Read the model definition and answer for the solid it produces. Units are mm, in the model's axes. A direction names the side the tool comes from. Coordinates: 2 decimals unless noted, no trailing zeros. Write each loop counter-clockwise with the first axis right and the second up, starting at its lowest first coordinate (ties: lowest second). Pieces come first, ordered by that corner, then holes. Notation, with made-up numbers: (76.5, -23.5) -> (89.5, -23.5) arc R25 cw to (89.5, 4.5) -> close; hole circle Ø8 at (38.5, -14). An arc over 180 degrees is marked (long way). Return JSON: item names as keys, results as strings.
from build123d import *

# Parameters (mm, degrees)
F0_W         = 51.3733290136
F0_H         = 51.9489385188
F1_DEPTH     = 63.5
F3_DEPTH     = 3.556
F4_T         = 2.54
F4_T3_DEPTH  = 13.7734491992
F4_T5_DEPTH  = 11.8834199066
F4_T7_DEPTH  = 11.0801313686
F4_T9_DEPTH  = 13.5809922736
F4_T11_DEPTH = 10.8262574938
F4_T13_DEPTH = 5.3370977176
F5_T1_DEPTH  = 76.2
F6_R         = 5.08


# Not quite as in the source:
# - a fillet or chamfer that OpenCascade refuses, or shapes differently, is made with other operations: its cross-section is extruded or revolved along the edge and cut away or added
# - a shell that OpenCascade refuses in one call is made with other operations: the cavity is built on its own and cut out


with BuildPart() as f1:
    # F0 (on Top) → F1 (new body)
    with BuildSketch(Plane.XY):
        with Locations((-25.6866645068, 25.9744692594)):
            Rectangle(F0_W, F0_H)
    extrude(amount=F1_DEPTH)

    # F2 (on Top) → F3 (join)
    with BuildSketch(Plane.XY):
        Polygon((-51.6957342625, 3.4017099533), (-51.6957342625, 0), (-45.3731976449, 0), (-45.3731976449, 6.8034199066), (-51.6957342625, 6.8034199066), align=None)
        Polygon((-45.3731976449, 43.2554893196), (-45.3731976449, 51.7564815932), (-51.6957342625, 51.9683584571), (-51.6957342625, 47.6119238883), (-51.6957342625, 43.2554893196), align=None)
    extrude(amount=-F3_DEPTH)

    # F4: shell of thickness 2.54, made by hand


with BuildPart() as f4_core1:
    # F4_t2: copy of F1
    add(f1.part)

    # the walls: a layer under each face that stays
    f4_faces = [f4_core1.faces().sort_by_distance(p)[0] for p in [
        (-25.8478671312, 0, 29.972),
        (-51.3733290136, 25.9744692594, 31.75),
        (-25.6866645068, 25.9744692594, 0),
        (-25.6866645068, 25.9744692594, 63.5),
        (-25.6866645068, 51.9489385188, 31.75),
        (-51.4059827792, 47.6119238883, 0),
        (-51.534531638, 3.4017099533, 0),
        (-51.6957342625, 3.4017099533, -1.778),
        (-45.3731976449, 3.4017099533, -1.778),
        (-48.5344659537, 3.4017099533, -3.556),
        (-48.5344659537, 6.8034199066, -1.778),
        (-48.5344659537, 43.2554893196, -1.778),
        (-45.3731976449, 47.5059854564, -1.778),
        (-48.5344659537, 51.8624200251, -1.778),
        (-51.6957342625, 47.6119238883, -1.778),
        (-48.5344659537, 47.6119238883, -3.556),
    ]]
    thicken(f4_faces, amount=-F4_T, mode=Mode.SUBTRACT)

    # F4_s4 → F4_t3 (cut)
    with BuildSketch(Plane.XZ.offset(-54.4889385188)):
        Polygon((-51.3987290136, 0.0254), (-48.8333290136, 0), (-48.8333290136, -2.54), (-51.3733290136, -2.54), align=None)
    extrude(amount=F4_T3_DEPTH, mode=Mode.SUBTRACT)

    # F4_s6 → F4_t5 (cut)
    with BuildSketch(Plane.XZ.offset(-9.3434199066)):
        Polygon((-51.3987290136, 0.0254), (-48.8333290136, 0), (-48.8333290136, -2.54), (-51.3733290136, -2.54), align=None)
        Polygon((-45.3477976449, -0.0254), (-45.3731976449, 2.54), (-47.9131976449, 2.54), (-47.9131976449, 0), align=None)
    extrude(amount=F4_T5_DEPTH, mode=Mode.SUBTRACT)

    # F4_s8 → F4_t7 (cut)
    with BuildSketch(Plane.YZ.offset(-53.9133290136)):
        Polygon((6.8288199066, -0.0254), (6.8034199066, 2.54), (4.2634199066, 2.54), (4.2634199066, 0), align=None)
        Polygon((43.2300893196, -0.0254), (43.2554893196, 2.54), (45.7954893196, 2.54), (45.7954893196, 0), align=None)
    extrude(amount=F4_T7_DEPTH, mode=Mode.SUBTRACT)

    # F4_s10 → F4_t9 (cut)
    with BuildSketch(Plane.XZ.offset(-54.2964815932)):
        Polygon((-45.3477976449, -0.0254), (-45.3731976449, 2.54), (-47.9131976449, 2.54), (-47.9131976449, 0), align=None)
    extrude(amount=F4_T9_DEPTH, mode=Mode.SUBTRACT)

    # F4_s12 → F4_t11 (cut)
    with BuildSketch(Plane(origin=(-44.5162101899, 1.4917991907, 0), x_dir=(0, 0, 1), z_dir=(-0.9994389665, 0.033492569, 0))):
        Polygon((-0.0254, 50.2331795219), (2.54, 50.2077795219), (2.54, 47.6677795219), (0, 47.6677795219), align=None)
    extrude(amount=F4_T11_DEPTH, mode=Mode.SUBTRACT)

    # F4_s14 → F4_t13 (cut)
    with BuildSketch(Plane.YZ.offset(-53.9133290136)):
        Polygon((51.9743385188, 0.0254), (49.4089385188, 0), (49.4089385188, -2.54), (51.9489385188, -2.54), align=None)
    extrude(amount=F4_T13_DEPTH, mode=Mode.SUBTRACT)


with BuildPart() as f1_1:
    add(f1.part)

    # what is left inside the walls is the cavity
    f4_cavity = [f4_core1.part.solids().sort_by_distance(p)[0] for p in [
        (-24.416665, 2.5654, 40.301333),
    ]]
    add(f4_cavity, mode=Mode.SUBTRACT)

    # F5: fillet of radius 5.08 on 2 edges, made by hand

    # F5_s2 → F5_t1 (cut)
    with BuildSketch(Plane.XY):
        with BuildLine():
            ThreePointArc((-46.2933290136, 0), (-49.885431462, 1.4878975516), (-51.3733290136, 5.08))
            Line((-51.3733290136, 5.08), (-51.3733290136, 0))
            Line((-51.3733290136, 0), (-46.2933290136, 0))
        make_face()
        with BuildLine():
            ThreePointArc((-51.3733290136, 46.8689385188), (-49.885431462, 50.4610409672), (-46.2933290136, 51.9489385188))
            Line((-46.2933290136, 51.9489385188), (-51.3733290136, 51.9489385188))
            Line((-51.3733290136, 51.9489385188), (-51.3733290136, 46.8689385188))
        make_face()
    extrude(amount=F5_T1_DEPTH, mode=Mode.SUBTRACT)

    # F6
    f6_edges = [f1_1.edges().sort_by_distance(p)[0] for p in [
        (-51.373329, 25.974469, 63.5),
        (-23.146665, 0, 63.5),
        (-23.146665, 51.948939, 63.5),
        (-49.885431, 50.461041, 63.5),
        (-49.885431, 1.487898, 63.5),
    ]]
    fillet(f6_edges, radius=F6_R)


solid = f1_1.part
1. Flat-ended cylindrical pins translate along their axes: pin 1 Ø14 at (x, z) = (-20, 27) entering from +Y; pin 2 Ø4 at (x, y) = (-33.5, 31) entering from -Z; pin 3 Ø0.5 at (x, z) = (-48.5, 1) entering from +Y. Find the tip coordinate at first contact, or state that the pin passes through.
Taken from the geometry:
{"pin 1": "stops at y = 51.95", "pin 2": "stops at z = 0", "pin 3": "stops at y = 51.56"}
2. The part is cut by section C-C (z = 44). Determine the outline of the cut face in (x, y).
Taken from the geometry:
{"outline": "(-51.37, 5.08) arc R5.08 ccw to (-46.29, 0) -> (0, 0) -> (0, 2.54) -> (-48.83, 2.54) -> (-48.83, 49.41) -> (0, 49.41) -> (0, 51.95) -> (-46.29, 51.95) arc R5.08 ccw to (-51.37, 46.87) -> close"}
3. The part is cut by section D-D (y = 48). Determine the outline of the cut face in (x, z).
Taken from the geometry:
{"outline": "(-51.7, -3.56) -> (-45.37, -3.56) -> (-45.37, 0) -> (0, 0) -> (0, 2.54) -> (-47.91, 2.54) -> (-47.91, -1.02) -> (-48.83, -1.02) -> (-48.83, 60.96) -> (0, 60.96) -> (0, 63.37) -> (-46.29, 63.37) arc R4.95 ccw to (-51.25, 58.42) -> (-51.25, 0) -> (-51.7, 0) -> close"}
4. A tool of negligible diameter and unlimited length cuts with its end or side. For faces 4 (the face through (-48, 6.803, -2)), 5 (the face through (-25, 49.409, 31)), 6 (the face through (-51, 2, 0)), 7 (the face through (-47.913, 48, 1)), from which of +Z, -Z, +X, -X, +Y, -Y can it reach the whole face along a straight path? Write none if from no direction.
Taken from the geometry:
{"face 4": "-Z, +X, -X", "face 5": "+X", "face 6": "+Z, -X, -Y", "face 7": "none"}
5. Consider L1, parallel to Y at x = -41, z = 34.5; L2, parallel to Z at x = -7.5, y = 39; L3, parallel to X at y = 27.5, z = 7. Determine where each line is inside the solid, lowest interval first.
Taken from the geometry:
{"L1": "y = 0 to 2.54, 49.41 to 51.95", "L2": "z = 0 to 2.54, 60.96 to 63.5", "L3": "x = -51.37 to -48.83"}
6. The part is cut by section B-B (y = 9). Determine the outline of the cut face in (x, z).
Taken from the geometry:
{"outline": "(-51.37, 0) -> (0, 0) -> (0, 2.54) -> (-48.83, 2.54) -> (-48.83, 60.96) -> (0, 60.96) -> (0, 63.5) -> (-46.29, 63.5) arc R5.08 ccw to (-51.37, 58.42) -> close"}
7. For a pull along Z with two mould halves and no side action, classify faces 1 (the face through (-25, 26, 2.54)), 2 (the face through (0, 1, 32)), 3 (the face through (-23, 26, 63.5)) as +Z half, -Z half, draft (parallel to the pull), parting line (faces both ways), or undercut.
Taken from the geometry:
{"face 1": "undercut", "face 2": "draft", "face 3": "+Z half"}
8. The part is cut by section A-A (x = -40.5). Determine the outline of the cut face in (y, z).
Taken from the geometry:
{"outline": "(0, 0) -> (51.95, 0) -> (51.95, 58.42) arc R5.08 ccw to (46.87, 63.5) -> (5.08, 63.5) arc R5.08 ccw to (0, 58.42) -> close; hole (2.54, 2.54) -> (49.41, 2.54) -> (49.41, 60.96) -> (2.54, 60.96) -> close"}
